Could you check a few things on this model? Use its own coordinates, in mm. Face numbers are marked on the shaded views. A direction names the side the tool comes from. Coordinates: 2 decimals unless noted, no trailing zeros. Write each loop counter-clockwise with the first axis right and the second up, starting at its lowest first coordinate (ties: lowest second). Pieces come first, ordered by that corner, then holes.
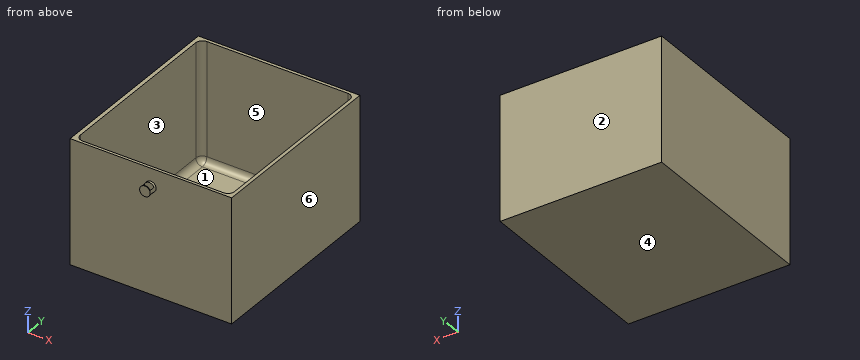
```python
from build123d import *

# Parameters (mm, degrees)
F0_W     = 125.476
F0_H     = 96.52
F1_DEPTH = 147.066
F2_W     = 119.730074
F2_H     = 142.576096
F3_DEPTH = 93.218
F4_R     = 4.07019
F5_DEPTH = 6.858
F6_W     = 7.457384
F6_H     = 3.801271
F7_DEPTH = 93.219
F8_W     = 7.396578
F8_H     = 3.085688
F9_DEPTH = 96.521
F10_R    = 5.08


with BuildPart() as f1:
    # F0 (on Front) → F1 (new body)
    with BuildSketch(Plane.XZ):
        Rectangle(F0_W, F0_H)
    extrude(amount=F1_DEPTH)

    # F2 (on face) → F3 (cut)
    with BuildSketch(Plane.XY.offset(48.26)):
        with Locations((0.211539, -73.679165)):
            Rectangle(F2_W, F2_H)
    extrude(amount=-F3_DEPTH, mode=Mode.SUBTRACT)

    # F4 (on face) → F5 (join)
    with BuildSketch(Plane.XZ.offset(147.066)):
        with Locations((0, 34.248885)):
            Circle(F4_R)
    extrude(amount=F5_DEPTH)

    # F6 (on face) → F7 (cut, through all)
    with BuildSketch(Plane.XY.offset(-44.958)):
        with Locations((0.002428, -151.50956)):
            Rectangle(F6_W, F6_H)
    extrude(amount=F7_DEPTH, mode=Mode.SUBTRACT)

    # F8 (on face) → F9 (cut, through all)
    with BuildSketch(Plane.XY.offset(48.26)):
        with Locations((-0.007179, -150.470339)):
            Rectangle(F8_W, F8_H)
    extrude(amount=-F9_DEPTH, mode=Mode.SUBTRACT)

    # F10
    f10_edges = [f1.edges().sort_by_distance(p)[0] for p in [
        (-59.653498, -144.967213, 1.651),
        (0.211539, -144.967213, -44.958),
        (-59.653498, -73.679165, -44.958),
        (60.076576, -73.679165, -44.958),
        (60.076576, -144.967213, 1.651),
        (0.211539, -2.391117, -44.958),
        (-59.653498, -2.391117, 1.651),
        (60.076576, -2.391117, 1.651),
    ]]
    fillet(f10_edges, radius=F10_R)


solid = f1.part
```
Item 1: I want a section at D-D, the plane x = 37. List the corners of the cut face in (y, z) for me, then the cut area to 3 significant figures.
Item 2: I want a section at A-A, the plane x = 0. List the corners of the cut face in (y, z) for me, then the cut area to 3 significant figures.
Item 3: Which directions (+Z, -Z, +X, -X, +Y, -Y) give clear straight access to the entire face, cutting with the end or side of a thin tool? Please do the marked faces 1 and 2.
Item 4: I want a section at B-B, the plane z = -34. List the corners of the cut face in (x, y) for me.
Item 5: If I drill on line 1 along Y through (x, z) = (-17, -27.5); line 2 along X through (y, z) = (-75, 24); line 3 along Z through (x, y) = (-55, -95.5), over which ranges is the centre line in solid material (lowest first)?
Item 6: Will these pins go through, and if not, where does the flat tip stop? pin 1 Ø1.5 at (x, z) = (35.5, -5.5) entering from -Y; pin 2 Ø6 at (x, y) = (-34.5, -27.5) entering from +Z; pin 3 Ø3.5 at (y, z) = (-151, 35) entering from -X.
Item 7: I want a section at C-C, the plane y = -90.5. List the corners of the cut face in (x, z) for me, then the cut area to 3 significant figures.
Item 8: If we mould it in two halves opening along X, with no side actions, what happens to the marked faces 3, 4, 5 and 6? For each: released by +X, released by -X, zero draft, split by the parting line, or undercut.
Taken from the geometry:
1. outline: (-147.07, -48.26) - (0, -48.26) - (0, 48.26) - (-2.39, 48.26) - (-2.39, -39.88) arc R5.08 cw to (-7.47, -44.96) - (-139.89, -44.96) arc R5.08 cw to (-144.97, -39.88) - (-144.97, 48.26) - (-147.07, 48.26) - close
1. area: 915 mm2
2. outline: (-153.92, 30.18) - (-153.41, 30.18) - (-153.41, 38.32) - (-153.92, 38.32) - close; (-148.93, 30.18) - (-147.07, 30.18) - (-147.07, -48.26) - (0, -48.26) - (0, 48.26) - (-2.39, 48.26) - (-2.39, -39.88) arc R5.08 cw to (-7.47, -44.96) - (-139.89, -44.96) arc R5.08 cw to (-144.97, -39.88) - (-144.97, 48.26) - (-147.07, 48.26) - (-147.07, 38.32) - (-148.93, 38.32) - close
2. area: 935 mm2
3. face 1: +Z
3. face 2: +Z, -Z, +X, -X, +Y
4. outline: (-62.74, -147.07) - (62.74, -147.07) - (62.74, 0) - (-62.74, 0) - close; hole (-59.65, -139.89) arc R5.08 ccw to (-54.57, -144.97) - (55, -144.97) arc R5.08 ccw to (60.08, -139.89) - (60.08, -7.47) arc R5.08 ccw to (55, -2.39) - (-54.57, -2.39) arc R5.08 ccw to (-59.65, -7.47) - close
5. line 1: y = -147.07 to -144.97, -2.39 to 0
5. line 2: x = -62.74 to -59.65, 60.08 to 62.74
5. line 3: z = -48.26 to -44.94
6. pin 1: stops at y = -147.07
6. pin 2: stops at z = -44.96
6. pin 3: stops at x = -4.07
7. outline: (-62.74, -48.26) - (62.74, -48.26) - (62.74, 48.26) - (60.08, 48.26) - (60.08, -39.88) arc R5.08 cw to (55, -44.96) - (-54.57, -44.96) arc R5.08 cw to (-59.65, -39.88) - (-59.65, 48.26) - (-62.74, 48.26) - close
7. area: 961 mm2
8. face 3: undercut
8. face 4: zero draft
8. face 5: undercut
8. face 6: released by +X
